Work out the finished part from the listing and answer in its coordinate system (mm). A direction names the side the tool comes from. Coordinates: 2 decimals unless noted, no trailing zeros. Loops run counter-clockwise (first coordinate to the right, second up) from the corner with the lowest first, then second, coordinate; pieces in that order, holes last. Notation, with made-up numbers: M 52,27.5 L 76,27.5 A15 ccw 76,38.5 Z; hole C 68,44.25 d7. An arc over 180 degrees is marked long. Write each question's results on one line, items separated by ' | '.
```python
from build123d import *

# Parameters (mm, degrees)
SKETCH1_W           = 20
SKETCH1_H           = 20
BOSS_EXTRUDE1_DEPTH = 11.89
SKETCH2_W           = 10
SKETCH2_H           = 10
CUT_EXTRUDE1_DEPTH  = 8
SKETCH101_R         = 2.15
CUT_EXTRUDE92_DEPTH = 6.825
SKETCH100_R         = 2.15
CUT_EXTRUDE93_DEPTH = 6.875
SKETCH99_R          = 2.15
CUT_EXTRUDE94_DEPTH = 4.825


with BuildPart() as part:
    # Sketch1 → Boss-Extrude1 (new body)
    with BuildSketch(Plane.XY):
        with Locations((10, 10)):
            Rectangle(SKETCH1_W, SKETCH1_H)
    extrude(amount=BOSS_EXTRUDE1_DEPTH)

    # Sketch2 → Cut-Extrude1 (cut)
    with BuildSketch(Plane.XY.offset(11.89)):
        with Locations((5, 5)):
            Rectangle(SKETCH2_W, SKETCH2_H)
    extrude(amount=-CUT_EXTRUDE1_DEPTH, mode=Mode.SUBTRACT)

    # Sketch101 → Cut-Extrude92 (cut)
    with BuildSketch(Plane(origin=(0, 20, 0), x_dir=(1, 0, 0), z_dir=(0, 1, 0))):
        with Locations((10, -5.945)):
            Circle(SKETCH101_R)
    extrude(amount=-CUT_EXTRUDE92_DEPTH, mode=Mode.SUBTRACT)

    # Sketch100 → Cut-Extrude93 (cut)
    with BuildSketch(Plane(origin=(20, 0, 0), x_dir=(0, 0, -1), z_dir=(1, 0, 0))):
        with Locations((-5.945, 10)):
            Circle(SKETCH100_R)
    extrude(amount=-CUT_EXTRUDE93_DEPTH, mode=Mode.SUBTRACT)

    # Sketch99 → Cut-Extrude94 (cut)
    with BuildSketch(Plane(origin=(0, 0, 0), x_dir=(-1, 0, 0), z_dir=(0, 0, -1))):
        with Locations((-15, 15)):
            Circle(SKETCH99_R)
    extrude(amount=-CUT_EXTRUDE94_DEPTH, mode=Mode.SUBTRACT)


solid = part.part
```
1) Find section B-B, the plane y = 15.5. Give the vertices of the cut face in (x, z) (3 decimals).
Check result:
outline: M 0,0 L 12.909,0 L 12.909,4.825 L 17.091,4.825 L 17.091,0 L 20,0 L 20,11.89 L 0,11.89 Z; hole C 10,5.945 d4.3
2) Straight lines are drawn through the part: probe 1 along Z at (x, y) = (10, 18.25) (3 decimals); probe 2 along Y at (x, z) = (15, 1.75); probe 3 along Y at (x, z) = (3, 4.5). For each, find the intervals that lie inside material, in ascending order. Write a range as [from, to].
Check result:
probe 1: [0, 3.795], [8.095, 11.89] | probe 2: [0, 12.85], [17.15, 20] | probe 3: [10, 20]
3) Find section A-A, the plane x = 17.5. Give the vertices of the cut face in (y, z) (3 decimals), and give its area (3 significant figures).
Check result:
outline: M 0,0 L 20,0 L 20,11.89 L 0,11.89 Z; hole C 10,5.945 d4.3 | area: 223 mm^2
4) Find section D-D, the plane z = 3.5. Give the vertices of the cut face in (x, y), and give its area (3 significant figures).
Check result:
outline: M 0,0 L 20,0 L 20,20 L 0,20 Z; hole C 15,15 d4.3 | area: 385 mm^2
5) Find section C-C, the plane x = 3.5. Give the vertices of the cut face in (y, z), and give its area (3 significant figures).
Check result:
outline: M 0,0 L 20,0 L 20,11.89 L 10,11.89 L 10,3.89 L 0,3.89 Z | area: 158 mm^2
6) Which of the six approach directions +Z, -Z, +X, -X, +Y, -Y give full straight-line access (tool end or side, diameter ignored) to faces 4 (the face through (14.01, 13.09, 2.38)), 5 (the face through (0, 12, 5)), 6 (the face through (9.72, 16.635, 3.813)), 7 (the face through (5, 5, 3.89)), 8 (the face through (16.61, 8.69, 7.65))?
Check result:
face 4: -Z | face 5: +Z, -Z, -X, +Y, -Y | face 6: +Y | face 7: +Z, -X, -Y | face 8: +X
7) For a pull along Z with two mould halves and no side action, classify faces 1 (the face through (5, 10, 8)), 2 (the face through (15, 15, 4.825)), 3 (the face through (10, 13.175, 6)) as released by +Z, released by -Z, zero draft, split by the parting line, or undercut.
Check result:
face 1: zero draft | face 2: released by -Z | face 3: undercut
8) Given pin 1 Ø1.3 at (x, y) = (14.5, 15) entering from -Z (3 decimals); pin 2 Ø6.5 at (x, z) = (6.5, 8.5) entering from -Y; pin 3 Ø6.5 at (y, z) = (6, 9) entering from -X, each flat-ended and moving along its own axis, determine where each tip first touches the part or whether it passes through.
Check result:
pin 1: z = 4.825 | pin 2: y = 10 | pin 3: x = 10
